Check sheet for the modelled part. Datum: model origin and axes. Units: mm. Face numbers are marked on the shaded views. A direction names the side the tool comes from. Give positions to 0.01 mm unless a question says otherwise; leave off trailing zeros. Order: outer loops, then holes, each group sorted by start corner. A loop starts at its lowest first (then second) coordinate and runs counter-clockwise, first axis right, second up.
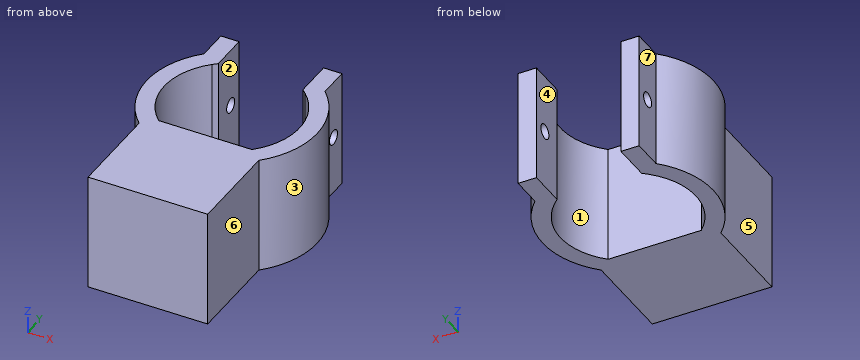
Autodesk Fusion 360 part; units mm, degrees
sketch "Sketch1" plane through (0, 0, 0) normal (0, 0, 1) x (1, 0, 0)
  arc A0 (7.9217, -8.3364) -> (7.9217, 8.3364) centre (0, 0) ccw
  line L0 (-7.1925, 15.5) -> (-10.2923, 15.5)
  line L1 (7.9217, -8.3364) -> (-7.9217, -8.3364)
  line L2 (7.1667, 15.5) -> (7.1667, 8.9938)
  line L3 (-10.2923, 15.5) -> (-10.2923, 10.2136)
  line L4 (10.2923, 15.5) -> (7.1667, 15.5)
  line L5 (7.9217, -8.3364) -> (-7.9217, -8.3364)
  line L6 (-10.2923, 15.5) -> (-10.2923, 10.2136)
  arc A1 (-10.2923, 10.2136) -> (-10.169, -10.3364) centre (0, 0) ccw
  line L7 (-7.1925, 15.5) -> (-7.1925, 8.9732)
  line L8 (10.2923, 10.2136) -> (10.2923, 15.5)
  arc A2 (-7.9217, 8.3364) -> (-7.9217, -8.3364) centre (0, 0) ccw
  circle A3 centre (0, 0) radius 11.5
  line L9 (-7.1925, 15.5) -> (-10.2923, 15.5)
  line L10 (10.2923, 10.2136) -> (10.2923, 15.5)
  line L11 (10.2923, 15.5) -> (7.1667, 15.5)
  arc A4 (10.169, -10.3364) -> (10.2923, 10.2136) centre (0, 0) ccw
  line L12 (10.169, -10.3364) -> (10.169, -26.3364)
  line L13 (-10.169, -10.3364) -> (-10.169, -26.3364)
  line L14 (-10.169, -26.3364) -> (10.169, -26.3364)
  dimension "d1" = 16
  dimension "d2" = 16
extrude "Extrude1" add sketch "Sketch1" along normal blind 20 contours L1 L5 A3 | A0 L0 L2 L3 L4 L6 A1 L7 L8 A2 A3 L9 L10 L11 A4 L12 L13 L14
sketch "Sketch2" plane through (10.2923, 0, 0) normal (1, 0, 0) x (0, 1, 0)
  line L0 (10.2136, 0) -> (15.5, 0)
  line L1 (15.5, 0) -> (15.5, 20)
  line L2 (15.5, 20) -> (10.2136, 20)
  line L3 (10.2136, 20) -> (10.2136, 0)
  line L4 (10.2136, 20) -> (15.5, 0) construction
  line L5 (10.2136, 0) -> (15.5, 20) construction
  circle A0 centre (12.8568, 10) radius 1.25
  dimension "d5" = 2.5
extrude "Extrude2" cut sketch "Sketch2" against normal blind 21 contours A0
(1) Release check for a two-part mould opening along Y. For the marked faces 1, 2 and 3 record: released by +Y, released by -Y, zero draft, split by the parting line, or undercut.
(2) Thickness scan on L1, parallel to X at y = -0.5, z = 2; L2, parallel to Y at x = -3.5, z = 2.5; L3, parallel to X at y = -15, z = 1.25. Record the ranges inside material, lowest first.
(3) Sectioned sample at A-A (z = 10). Enter the section's corners in (x, y), plus the area to 3 significant figures.
(4) Sectioned sample at B-B (y = -14.5). Enter the section's corners in (x, z).
(5) Tool access check on the marked faces 4, 5, 6 and 7. Record the directions out of +Z, -Z, +X, -X, +Y, -Y that give a thin tool (end or side, any length) a straight path to the whole face; none if there is none.
(6) Go/stop test with flat-tipped pins: P1, Ø1.6, axis at y = 14, z = 9, coming from the +X side; P2, Ø3, axis at x = 3, z = 16.5, coming from the +Y side; P3, Ø6, axis at x = -3.5, y = 9.5, coming from the +Z side; P4, Ø8, axis at y = -22, z = 13.5, coming from the -X side. Record where each tip stops, or that it passes through.
(7) Sectioned sample at D-D (z = 14.75). Enter the section's corners in (x, y).
(8) Sectioned sample at C-C (x = -6.25). Enter the section's corners in (y, z), plus the area to 3 significant figures.
Values follow:
1. face 1: undercut
1. face 2: zero draft
1. face 3: split by the parting line
2. L1: x = -14.49 to -11.49, 11.49 to 14.49
2. L2: y = -26.34 to -8.34
2. L3: x = -10.17 to 10.17
3. outline: (-10.29, 10.21) arc R14.5 ccw to (-10.17, -10.34) - (-10.17, -26.34) - (10.17, -26.34) - (10.17, -10.34) arc R14.5 ccw to (10.29, 10.21) - (10.29, 11.61) - (7.17, 11.61) - (7.17, 8.99) arc R11.5 cw to (7.92, -8.34) - (-7.92, -8.34) arc R11.5 cw to (-7.92, 8.34) arc R11.5 cw to (-7.19, 8.97) - (-7.19, 11.61) - (-10.29, 11.61) - close; (-10.29, 14.11) - (-7.19, 14.11) - (-7.19, 15.5) - (-10.29, 15.5) - close; (7.17, 14.11) - (10.29, 14.11) - (10.29, 15.5) - (7.17, 15.5) - close
3. area: 510 mm2
4. outline: (-10.17, 0) - (10.17, 0) - (10.17, 20) - (-10.17, 20) - close
5. face 4: +Z, -Z, +Y
5. face 5: +Z, -Z, -X, -Y
5. face 6: +Z, -Z, +X, -Y
5. face 7: +Z, -Z, -X, +Y
6. P1: stops at x = 10.29
6. P2: stops at y = -8.34
6. P3: passes through
6. P4: stops at x = -10.17
7. outline: (-10.29, 10.21) arc R14.5 ccw to (-10.17, -10.34) - (-10.17, -26.34) - (10.17, -26.34) - (10.17, -10.34) arc R14.5 ccw to (10.29, 10.21) - (10.29, 15.5) - (7.17, 15.5) - (7.17, 8.99) arc R11.5 cw to (7.92, -8.34) - (-7.92, -8.34) arc R11.5 cw to (-7.92, 8.34) arc R11.5 cw to (-7.19, 8.97) - (-7.19, 15.5) - (-10.29, 15.5) - close
8. outline: (-26.34, 0) - (-8.34, 0) - (-8.34, 20) - (-26.34, 20) - close
8. area: 360 mm2
